The model under review builds one solid part; all positions refer to its coordinate system, in mm. Round coordinates to 2 decimals unless told otherwise and drop trailing zeros. Order: outer loops, then holes, each group sorted by start corner. A loop starts at its lowest first (then second) coordinate and runs counter-clockwise, first axis right, second up.
```python
from build123d import *

# Parameters (mm, degrees)
SKETCH1_R           = 2.0828
BOSS_EXTRUDE1_DEPTH = 3.175
FILLET1_R           = 1.5875
FILLET2_R           = 3.175
FILLET3_R           = 1.5875


with BuildPart() as part:
    # Sketch1 → Boss-Extrude1 (new body)
    with BuildSketch(Plane(origin=(0, 0, 0), x_dir=(1, 0, 0), z_dir=(0, 1, 0))):
        with BuildLine():
            Line((26.924, -25.4), (-26.924, -25.4))
            Line((-26.924, -25.4), (-26.924, -28.575))
            Line((-26.924, -28.575), (-46.228, -28.575))
            Line((-46.228, -28.575), (-74.803, -28.575))
            Line((-74.803, -28.575), (-74.803, 28.575))
            Line((-74.803, 28.575), (-46.228, 28.575))
            Line((-46.228, 28.575), (-26.924, 28.575))
            Line((-26.924, 28.575), (-26.924, 25.4))
            Line((-26.924, 25.4), (26.924, 25.4))
            Line((26.924, 25.4), (26.924, 31.75))
            Line((26.924, 31.75), (52.324, 31.75))
            Line((52.324, 31.75), (62.607581289, 63.240132856))
            ThreePointArc((62.607581289, 63.240132856), (72.010560326, 69.32064995), (80.585058538, 62.118797179))
            Line((80.585058538, 62.118797179), (87.884, 31.75))
            Line((87.884, 31.75), (138.684, 31.75))
            Line((138.684, 31.75), (138.684, -31.75))
            Line((138.684, -31.75), (87.884, -31.75))
            Line((87.884, -31.75), (80.585058538, -62.118797179))
            ThreePointArc((80.585058538, -62.118797179), (72.010560326, -69.32064995), (62.607581289, -63.240132856))
            Line((62.607581289, -63.240132856), (52.324, -31.75))
            Line((52.324, -31.75), (26.924, -31.75))
            Line((26.924, -31.75), (26.924, -25.4))
        make_face()
        with Locations(Location((71.4240126, 59.9169998, 0), (0, 0, 270))):
            Circle(SKETCH1_R, mode=Mode.SUBTRACT)
        with Locations(Location((71.4240126, -59.9169998, 0), (0, 0, 90))):
            Circle(SKETCH1_R, mode=Mode.SUBTRACT)
        with BuildLine():
            Line((77.7740126, 31.75), (65.0740126, 31.75))
            Line((65.0740126, 31.75), (69.141994412, 44.206875103))
            ThreePointArc((69.141994412, 44.206875103), (71.4240126, 44.0419998), (73.706030788, 44.206875103))
            Line((73.706030788, 44.206875103), (77.7740126, 31.75))
        make_face(mode=Mode.SUBTRACT)
        with BuildLine():
            Line((77.7740126, -31.75), (73.706030788, -44.206875103))
            ThreePointArc((73.706030788, -44.206875103), (71.4240126, -44.0419998), (69.141994412, -44.206875103))
            Line((69.141994412, -44.206875103), (65.0740126, -31.75))
            Line((65.0740126, -31.75), (77.7740126, -31.75))
        make_face(mode=Mode.SUBTRACT)
    extrude(amount=BOSS_EXTRUDE1_DEPTH)

    # Fillet1
    fillet1_edges = [part.edges().sort_by_distance(p)[0] for p in [
        (69.141994412, 1.5875, 44.206875103),
        (73.706030788, 1.5875, 44.206875103),
        (69.141994412, 1.5875, -44.206875103),
        (73.706030788, 1.5875, -44.206875103),
    ]]
    fillet(fillet1_edges, radius=FILLET1_R)

    # Fillet2
    fillet2_edges = [part.edges().sort_by_distance(p)[0] for p in [
        (77.7740126, 1.5875, 31.75),
        (65.0740126, 1.5875, 31.75),
        (65.0740126, 1.5875, -31.75),
        (77.7740126, 1.5875, -31.75),
    ]]
    fillet(fillet2_edges, radius=FILLET2_R)

    # Fillet3
    fillet3_edges = [part.edges().sort_by_distance(p)[0] for p in [
        (138.684, 1.5875, -31.75),
        (138.684, 1.5875, 31.75),
    ]]
    fillet(fillet3_edges, radius=FILLET3_R)


solid = part.part
```
(1) Consider section B-B (y = 0.8). State how many separate pieces and enclosed holes the cut face has, and give its area (3 significant figures).
Data:
separate pieces: 1
enclosed holes: 4
area: 14,200 mm2
(2) To check wall thickness, follow probe 1 along Z at (x, y) = (8, 1.85); probe 2 along Z at (x, y) = (107.5, 0.4); probe 3 along X at (y, z) = (0.9, -37.5). State the ranges of each line that lie inside material, in increasing order.
Data:
probe 1: z = -25.4 to 25.4
probe 2: z = -31.75 to 31.75
probe 3: x = 54.2 to 66.95, 75.9 to 86.5
(3) Consider section A-A (x = -22). Write out the cut boundary in (y, z) (3 decimals).
Data:
outline: (0, -25.4) - (3.175, -25.4) - (3.175, 25.4) - (0, 25.4) - close
(4) Insertion check: pin 1 (1 mm diameter, centred on x = 70.5, y = 1, fed in from +Z); pin 2 (5.5 mm diameter, centred on x = 71.42, z = -59.92, fed in from +Y) (3 decimals); pin 3 (1.6 mm diameter, centred on x = 114, y = 1.5, fed in from +Z). Each pin has a flat end and moves straight along its axis. Give the tip position at first contact, or say it passes through.
Data:
pin 1: stops at z = 69.33
pin 2: stops at y = 3.175
pin 3: stops at z = 31.75
(5) Draft analysis for pull direction Z (two halves, no side actions). For faces 1 (the flat face through (57.54, 1.57, 47.72)), 2 (the cylindrical face through (71.84, 1.57, -69.33)), 3 (the cylindrical face through (70.016, 1.565, 61.452)), state which applies: pulls with the +Z half, pulls with the -Z half, needs draft (parallel to the pull), parting line crosses it, or undercut.
Data:
face 1: pulls with the +Z half
face 2: pulls with the -Z half
face 3: undercut
(6) Consider section C-C (x = 31). Write out the cut boundary in (y, z) (3 decimals).
Data:
outline: (0, -31.75) - (3.175, -31.75) - (3.175, 31.75) - (0, 31.75) - close
